from build123d import *

# Parameters (mm, degrees)
F0_W     = 92
F0_H     = 58
F0_W_2   = 84
F0_H_2   = 50
F0_R     = 5
F1_DEPTH = 4
F2_DEPTH = 25
F3_DEPTH = 3
F5_DEPTH = 4
F6_R     = 4.1
F7_DEPTH = 4
F9_D     = 4.1


with BuildPart() as f1:
    # F0 (on Top) → F1 (new body)
    with BuildSketch(Plane.XY):
        with Locations((27, -15)):
            Rectangle(F0_W, F0_H)
        with Locations((27, -15)):
            Rectangle(F0_W_2, F0_H_2, mode=Mode.SUBTRACT)
        with Locations((27, -15)):
            Rectangle(F0_W_2, F0_H_2)
        with Locations((11, -27)):
            Circle(F0_R, mode=Mode.SUBTRACT)
        with Locations((35, -3)):
            Circle(F0_R, mode=Mode.SUBTRACT)
        with Locations((11, -27)):
            Circle(F0_R)
        with Locations((35, -3)):
            Circle(F0_R)
    extrude(amount=-F1_DEPTH)

    # F0 (on Top) → F2 (join)
    with BuildSketch(Plane.XY):
        with Locations((27, -15)):
            Rectangle(F0_W, F0_H)
        with Locations((27, -15)):
            Rectangle(F0_W_2, F0_H_2, mode=Mode.SUBTRACT)
    extrude(amount=F2_DEPTH)

    # F0 (on Top) → F3 (join)
    with BuildSketch(Plane.XY):
        with Locations((35, -3)):
            Circle(F0_R)
        with Locations((11, -27)):
            Circle(F0_R)
    extrude(amount=F3_DEPTH)

    # F4 (on face) → F5 (cut, through all)
    with BuildSketch(Plane.YZ.offset(73)):
        with BuildLine():
            Line((-28.704477, 8.884444), (-28.704477, 10.884444))
            ThreePointArc((-28.704477, 10.884444), (-29.954477, 17.134444), (-31.204477, 10.884444))
            Line((-31.204477, 10.884444), (-31.204477, 8.884444))
            ThreePointArc((-31.204477, 8.884444), (-29.954477, 7.634444), (-28.704477, 8.884444))
        make_face()
        with BuildLine():
            Line((-12.469048, 17.384444), (-16.342031, 17.384444))
            ThreePointArc((-16.342031, 17.384444), (-18.40554, 13.884444), (-16.342031, 10.384444))
            Line((-16.342031, 10.384444), (-12.469048, 10.384444))
            ThreePointArc((-12.469048, 10.384444), (-10.40554, 13.884444), (-12.469048, 17.384444))
        make_face()
        with BuildLine():
            Line((-2.4822, 10.384444), (1.390783, 10.384444))
            ThreePointArc((1.390783, 10.384444), (3.454292, 13.884444), (1.390783, 17.384444))
            Line((1.390783, 17.384444), (-2.4822, 17.384444))
            ThreePointArc((-2.4822, 17.384444), (-4.545708, 13.884444), (-2.4822, 10.384444))
        make_face()
    extrude(amount=-F5_DEPTH, mode=Mode.SUBTRACT)

    # F6 (on face) → F7 (cut, through all)
    with BuildSketch(Plane(origin=(-19, 0, 0), x_dir=(0, -1, 0), z_dir=(-1, 0, 0))):
        with Locations((1.185031, 13.089023)):
            Circle(F6_R)
        with BuildLine():
            Line((18.530197, 5.589023), (18.530197, 9.816409))
            ThreePointArc((18.530197, 9.816409), (17.030197, 16.689023), (15.530197, 9.816409))
            Line((15.530197, 9.816409), (15.530197, 5.589023))
            ThreePointArc((15.530197, 5.589023), (17.030197, 4.089023), (18.530197, 5.589023))
        make_face()
    extrude(amount=-F7_DEPTH, mode=Mode.SUBTRACT)

    # F9 (through all)
    with Locations(Plane.XY.offset(3)):
        with Locations((35, -3), (11, -27)):
            Hole(F9_D / 2)


solid = f1.part
Model file for the job. Use its own axes, mm. A direction names the side the tool comes from. Round coordinates to 2 decimals unless told otherwise and drop trailing zeros. Loops run counter-clockwise (first coordinate to the right, second up) from the corner with the lowest first, then second, coordinate; pieces in that order, holes last.
1. Drop flat-ended pins along their axis: P1, Ø5, axis at y = -1.19, z = 13.09, coming from the +X side; P2, Ø3, axis at x = 58, y = -32.5, coming from the +Z side; P3, Ø6, axis at y = -17.03, z = 13.09, coming from the -X side; P4, Ø3, axis at x = 12.5, y = -28, coming from the +Z side. Give the stop position or say it passes through.
Check values:
P1: passes through
P2: stops at z = 0
P3: stops at x = 69
P4: stops at z = 3
2. Band-saw the part on D-D, the plane y = -36. List the corners of the cut face in (x, z), and give its area (3 significant figures).
Check values:
outline: (-19, -4) - (73, -4) - (73, 25) - (69, 25) - (69, 0) - (-15, 0) - (-15, 25) - (-19, 25) - close
area: 568 mm2
3. Band-saw the part on B-B, the plane y = -7. List the corners of the cut face in (x, z), and give its area (3 significant figures).
Check values:
outline: (-19, -4) - (73, -4) - (73, 25) - (69, 25) - (69, 0) - (38, 0) - (38, 3) - (32, 3) - (32, 0) - (-15, 0) - (-15, 25) - (-19, 25) - close
area: 586 mm2
4. Mould opens along Z. For faces 4 (the cylindrical face through (12.5, -25.6, -0.5)), 5 (the cylindrical face through (-17.028, -17.167, 16.686)), 6 (the flat face through (26, -15, 0)), 7 (the flat face through (-17, -15.53, 8)) say: +Z half, -Z half, draft (parallel to the pull), parting line (faces both ways), or undercut.
Check values:
face 4: draft
face 5: undercut
face 6: +Z half
face 7: undercut
5. Tool access for faces 1 (the cylindrical face through (30, -3, 1)), 2 (the cylindrical face through (-17.03, -17, 4.09)), 3 (the cylindrical face through (71.028, -29.982, 7.635)): list every direction of +Z, -Z, +X, -X, +Y, -Y with a clear straight run to the whole face (end or side of a thin tool).
Check values:
face 1: +Z
face 2: -X
face 3: +X
6. Band-saw the part on C-C, the plane z = 15.25. List the corners of the cut face in (x, y), and give its area (3 significant figures).
Check values:
outline: (-19, -44) - (73, -44) - (73, -32.9) - (69, -32.9) - (69, -40) - (-15, -40) - (-15, -19.91) - (-19, -19.91) - close; (-19, -14.15) - (-15, -14.15) - (-15, -4.67) - (-19, -4.67) - close; (-19, 2.3) - (-15, 2.3) - (-15, 10) - (69, 10) - (69, 3.21) - (73, 3.21) - (73, 14) - (-19, 14) - close; (69, -27.01) - (73, -27.01) - (73, -18.17) - (69, -18.17) - close; (69, -10.65) - (73, -10.65) - (73, -4.31) - (69, -4.31) - close
area: 1,000 mm2
7. Band-saw the part on A-A, the plane x = 11. List the corners of the cut face in (y, z), and give its area (3 significant figures).
Check values:
outline: (-44, -4) - (-29.05, -4) - (-29.05, 3) - (-32, 3) - (-32, 0) - (-40, 0) - (-40, 25) - (-44, 25) - close; (-24.95, -4) - (14, -4) - (14, 25) - (10, 25) - (10, 0) - (-22, 0) - (-22, 3) - (-24.95, 3) - close
area: 433 mm2
8. Wall check: probe 1 along Y at (x, z) = (16.5, 17); probe 2 along X at (y, z) = (7, 0.5); probe 3 along Y at (x, z) = (11, -2.5). Give the ranges that are in metal, low to high.
Check values:
probe 1: y = -44 to -40, 10 to 14
probe 2: x = -19 to -15, 69 to 73
probe 3: y = -44 to -29.05, -24.95 to 14
